Design review of the part built by this model. Coordinates are the model's own, in mm. A direction names the side the tool comes from. Round coordinates to 2 decimals unless told otherwise and drop trailing zeros. Order: outer loops, then holes, each group sorted by start corner. A loop starts at its lowest first (then second) coordinate and runs counter-clockwise, first axis right, second up. Notation, with made-up numbers: M 20,48.25 L 45,48.25 A26 cw 45,77.25 Z; hole C -40,6 d10. An arc over 180 degrees is marked long. Write each question's results on one line, items separated by ' | '. Start each with the question number.
Item 1: Clearance check with flat-ended pins moving along their axes: pin 1 (1.2 mm diameter, centred on x = -34.5, z = 15, fed in from +Y); pin 2 (1.5 mm diameter, centred on x = 11, z = -2, fed in from +Y). State where each tip first meets the part, or that it passes through.
Item 2: The part is to be moulded in two halves that separate along Z. For faces 3 (the cylindrical face through (36, 2, 17)), 4 (the cylindrical face through (-33.66, 1.52, -14.46)), 5 (the flat face through (-37, 1, 0)), say which applies: +Z half, -Z half, draft (parallel to the pull), parting line (faces both ways), or undercut.
Item 3: Take a section at B-B, the plane x = -19. Write out the cut boundary in (y, z).
Item 4: Take a section at A-A, the plane z = 3.5. Write out the cut boundary in (x, y), plus the area to 3 significant figures.
Item 5: Machinability: for faces 1 (the flat face through (0, 2, 0)), 2 (the cylindrical face through (33.66, 1.52, 14.46)), which of the approach directions +Z, -Z, +X, -X, +Y, -Y give a long, thin tool a straight path to every point of the face, cutting with its end or side? Answer none if there is none.
Item 6: Wall thickness on line 1 (Z direction, x = 34.5, y = 1); line 2 (X direction, y = 0.65, z = 15); line 3 (X direction, y = 2.7, z = -15): over which ranges is each line inside the solid? List them lowest first. Write a range as [from, to].
```python
from build123d import *

# Parameters (mm, degrees)
SZKIC1_W                    = 74
SZKIC1_H                    = 35
DODANIE_WYCI_GNI_CIE1_DEPTH = 3
SZKIC2_W                    = 53
SZKIC2_H                    = 33
WYTNIJ_WYCI_GNI_CIE1_DEPTH  = 1
SZKIC4_R                    = 1
WYTNIJ_WYCI_GNI_CIE2_DEPTH  = 42.039615008
ZAOKR_GLENIE1_R             = 2.5
LUSTRO2_COPY_1_SKETCH_R     = 1
LUSTRO2_COPY_1_DEPTH        = 42.039615008


with BuildPart() as part:
    # Szkic1 → Dodanie-wyciągnięcie1 (new body)
    with BuildSketch(Plane(origin=(0, 0, 0), x_dir=(1, 0, 0), z_dir=(0, 1, 0))):
        Rectangle(SZKIC1_W, SZKIC1_H)
    extrude(amount=DODANIE_WYCI_GNI_CIE1_DEPTH)

    # Szkic2 → Wytnij-wyciągnięcie1 (cut)
    with BuildSketch(Plane(origin=(0, 3, 0), x_dir=(1, 0, 0), z_dir=(0, 1, 0))):
        Rectangle(SZKIC2_W, SZKIC2_H)
    extrude(amount=-WYTNIJ_WYCI_GNI_CIE1_DEPTH, mode=Mode.SUBTRACT)

    # Szkic4 → Wytnij-wyciągnięcie2 (cut, through all)
    with BuildSketch(Plane(origin=(0, 3, 0), x_dir=(1, 0, 0), z_dir=(0, 1, 0))):
        with Locations(Location((-34.5, 15, 0), (0, 0, 270))):
            Circle(SZKIC4_R)
    wytnij_wyci_gni_cie2 = extrude(amount=-WYTNIJ_WYCI_GNI_CIE2_DEPTH, mode=Mode.SUBTRACT)

    # Zaokrąglenie1
    zaokr_glenie1_edges = [part.edges().sort_by_distance(p)[0] for p in [
        (37, 1.5, 17.5),
        (-37, 1.5, 17.5),
        (-37, 1.5, -17.5),
        (37, 1.5, -17.5),
    ]]
    fillet(zaokr_glenie1_edges, radius=ZAOKR_GLENIE1_R)

    # Lustro1: Wytnij-wyciągnięcie2 across plane
    add(wytnij_wyci_gni_cie2.mirror(Plane.XY), mode=Mode.SUBTRACT)

    # Lustro2: Wytnij-wyciągnięcie2 across plane
    add(wytnij_wyci_gni_cie2.mirror(Plane(origin=(0, 0, 0), x_dir=(0, 0, 1), z_dir=(1, 0, 0))), mode=Mode.SUBTRACT)

    # Lustro2 copy 1 sketch → Lustro2 copy 1 (cut, through all)
    with BuildSketch(Plane(origin=(0, 3, 0), x_dir=(-1, 0, 0), z_dir=(0, 1, 0))):
        with Locations(Location((-34.5, 15, 0), (0, 0, 270))):
            Circle(LUSTRO2_COPY_1_SKETCH_R)
    extrude(amount=-LUSTRO2_COPY_1_DEPTH, mode=Mode.SUBTRACT)


solid = part.part
```
Results list:
1) pin 1: through | pin 2: y = 2
2) face 3: +Z half | face 4: undercut | face 5: draft
3) outline: M 0,-17.5 L 3,-17.5 L 3,-16.5 L 2,-16.5 L 2,16.5 L 3,16.5 L 3,17.5 L 0,17.5 Z
4) outline: M -37,0 L 37,0 L 37,3 L 26.5,3 L 26.5,2 L -26.5,2 L -26.5,3 L -37,3 Z | area: 169 mm²
5) face 1: +Y | face 2: +Y, -Y
6) line 1: [-17.5, -16], [-14, 14], [16, 17.5] | line 2: [-37, -35.5], [-33.5, 33.5], [35.5, 37] | line 3: [-37, -35.5], [-33.5, -26.5], [26.5, 33.5], [35.5, 37]
